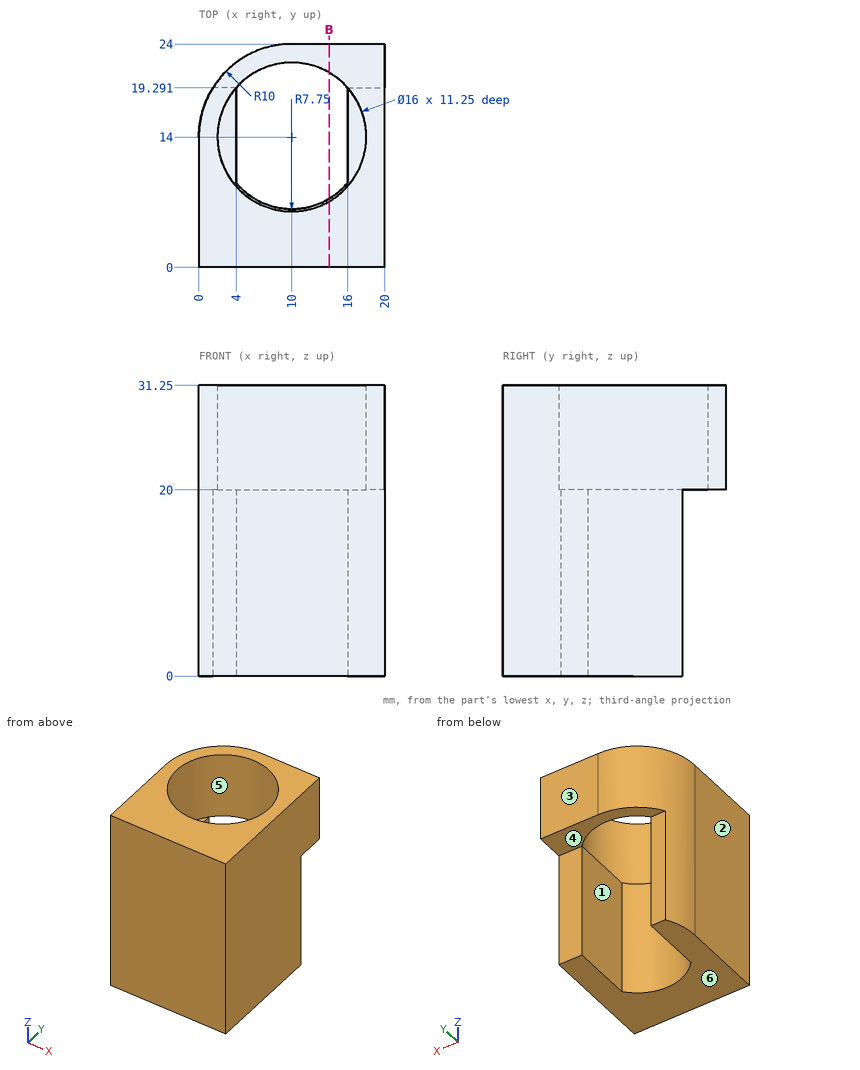
Drawing for the job (mm, zero at the part's lowest x, y, z). A direction names the side the tool comes from. Round coordinates to 2 decimals unless told otherwise and drop trailing zeros. Write each loop counter-clockwise with the first axis right and the second up, starting at its lowest first coordinate (ties: lowest second). Pieces come first, ordered by that corner, then holes. Notation, with made-up numbers: M -29,1.5 L 16,1.5 A16 cw 16,18.5 Z; hole C -25,-20.75 d2. An arc over 180 degrees is marked long. Answer as a JSON object with one key per item and string values. Group by question number.
(1) Flat gauge pins, fed straight in: pin 1 (6 mm diameter, centred on x = 7.5, z = 9.5, fed in from +Y); pin 2 (4 mm diameter, centred on x = 7, y = 10.5, fed in from +Z); pin 3 (2 mm diameter, centred on x = 2.5, z = 7, fed in from +Y); pin 4 (4 mm diameter, centred on x = 8.5, y = 21, fed in from -Z). Where does each tip first touch, or does it go through?
(2) Which spindle directions (+Z, -Z, +X, -X, +Y, -Y) get a long thin tool onto all of the face, cutting with end or side? Do the marked faces 4, 5 and 6. Say none if no direction does.
(3) Mould opens along X. For the marked faces 1, 2 and 3 say: pulls with the +X half, pulls with the -X half, needs draft (parallel to the pull), parting line crosses it, or undercut.
(4) Drill centre lines: L1, parallel to X at y = 14, z = 26; L2, parallel to Y at x = 10, z = 23; L3, parallel to X at y = 13.5, z = 6.5. Where is each one in solid material? Low to high.
(5) Cut at B-B (x = 14). Give the cut face in (y, z), and give its area (3 significant figures).
Responses:
{
 "1": {"pin 1": "stops at y = 8.54", "pin 2": "passes through", "pin 3": "stops at y = 19.29", "pin 4": "stops at z = 20"},
 "2": {"face 4": "-Z, +X, -X, +Y", "face 5": "+Z", "face 6": "-Z, +X, -X, +Y, -Y"},
 "3": {"face 1": "undercut", "face 2": "pulls with the -X half", "face 3": "needs draft"},
 "4": {"L1": "x = 0 to 2, 18 to 20", "L2": "y = 0 to 6, 22 to 24", "L3": "x = 0 to 4, 16 to 20"},
 "5": {"outline": "M 0,0 L 7.36,0 L 7.36,20 L 7.07,20 L 7.07,31.25 L 0,31.25 Z; M 20.93,20 L 24,20 L 24,31.25 L 20.93,31.25 Z", "area": "261 mm2"}
}
